Verification items for the finished model (mm, model axes). Face numbers are marked on the shaded views. Round coordinates to 2 decimals unless told otherwise and drop trailing zeros. Write each loop counter-clockwise with the first axis right and the second up, starting at its lowest first coordinate (ties: lowest second). Pieces come first, ordered by that corner, then holes.
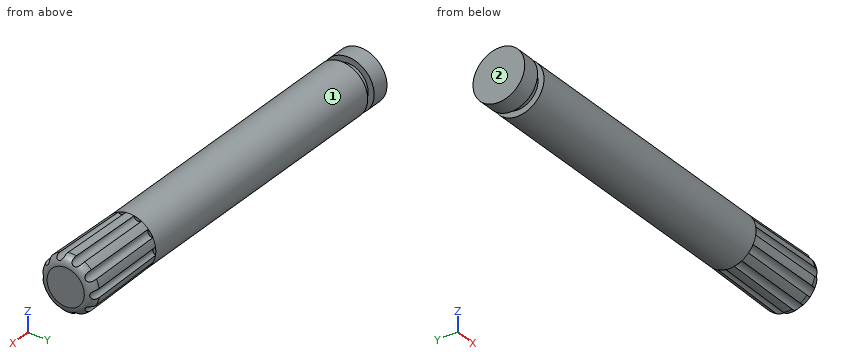
from build123d import *

# Parameters (mm, degrees)
SKETCH1_R                = 1.5
EXTRUDE1_DEPTH           = 18
EXTRUDE1_OTHER_WAY_DEPTH = 5
EXTRUDE1_OTHER_WAY_TAPER = -1
FILLET1_R                = 0.5
SKETCH2_R                = 0.25
CUT_EXTRUDE1_DEPTH       = 5
CIRPATTERN1_COUNT        = 10
SKETCH3_W                = 0.5
SKETCH3_H                = 0.930924855


with BuildPart() as part:
    # Sketch1 → Extrude1 (new body)
    with BuildSketch(Plane(origin=(0, 0, 0), x_dir=(0, 0, -1), z_dir=(1, 0, 0))):
        Circle(SKETCH1_R)
    extrude(amount=-EXTRUDE1_DEPTH)

    # Sketch1 → Extrude1 other way (add)
    with BuildSketch(Plane(origin=(0, 0, 0), x_dir=(0, 0, -1), z_dir=(1, 0, 0))):
        Circle(SKETCH1_R)
    extrude(amount=EXTRUDE1_OTHER_WAY_DEPTH, taper=EXTRUDE1_OTHER_WAY_TAPER)

    # Fillet1
    fillet1_edges = [part.edges().sort_by_distance(p)[0] for p in [
        (5, 0, 1.587275325),
    ]]
    fillet(fillet1_edges, radius=FILLET1_R)

    # Sketch2 → Cut-Extrude1 (cut)
    with BuildSketch(Plane(origin=(5, 0, 0), x_dir=(0, 0, -1), z_dir=(1, 0, 0))):
        with Locations((0, 1.587275325)):
            Circle(SKETCH2_R)
    cut_extrude1 = extrude(amount=-CUT_EXTRUDE1_DEPTH, mode=Mode.SUBTRACT)

    # CirPattern1: Cut-Extrude1 ×10 about axis
    cirpattern1_axis = Axis((0, 0, 0), (1, 0, 0))
    for i in range(1, CIRPATTERN1_COUNT):
        add(cut_extrude1.rotate(cirpattern1_axis, i * 360 / CIRPATTERN1_COUNT), mode=Mode.SUBTRACT)

    # Sketch3 → Cut-Revolve2 (revolve, cut)
    with BuildSketch(Plane.XY):
        with Locations((-16.75, 1.615462428)):
            Rectangle(SKETCH3_W, SKETCH3_H)
    revolve(axis=Axis((-18, 0, 0), (1, 0, 0)), mode=Mode.SUBTRACT)


solid = part.part
Q1. Sectioned sample at A-A (z = 0). Enter the section's corners in (x, y).
Recorded:
outline: (-18, -1.5) - (-17, -1.5) - (-17, -1.15) - (-16.5, -1.15) - (-16.5, -1.5) - (0, -1.5) - (0, -1.34) - (4.93, -1.34) arc R0.5 ccw to (5, -1.08) - (5, 1.08) arc R0.5 ccw to (4.93, 1.34) - (0, 1.34) - (0, 1.5) - (-16.5, 1.5) - (-16.5, 1.15) - (-17, 1.15) - (-17, 1.5) - (-18, 1.5) - close
Q2. Release check for a two-part mould opening along Y. For the marked faces 1 and 2 record: released by +Y, released by -Y, zero draft, split by the parting line, or undercut.
Recorded:
face 1: split by the parting line
face 2: zero draft
Q3. Sectioned sample at B-B (x = 3.25). Enter the section's corners in (y, z), plus the area to 3 significant figures.
Recorded:
outline: (-1.54, -0.24) arc R1.56 ccw to (-1.39, -0.71) arc R0.25 cw to (-1.1, -1.1) arc R1.56 ccw to (-0.71, -1.39) arc R0.25 cw to (-0.24, -1.54) arc R1.56 ccw to (0.24, -1.54) arc R0.25 cw to (0.71, -1.39) arc R1.56 ccw to (1.1, -1.1) arc R0.25 cw to (1.39, -0.71) arc R1.56 ccw to (1.54, -0.24) arc R0.25 cw to (1.54, 0.24) arc R1.56 ccw to (1.39, 0.71) arc R0.25 cw to (1.1, 1.1) arc R1.56 ccw to (0.71, 1.39) arc R0.25 cw to (0.24, 1.54) arc R1.56 ccw to (-0.24, 1.54) arc R0.25 cw to (-0.71, 1.39) arc R1.56 ccw to (-1.1, 1.1) arc R0.25 cw to (-1.39, 0.71) arc R1.56 ccw to (-1.54, 0.24) arc R0.25 cw to start
area: 6.82 mm2
Q4. Material ranges on line 1 along Z through (x, y) = (2.5, -0.5); line 2 along Y through (x, z) = (0.5, -1.1); line 3 along Y through (x, z) = (3, -0.65), recorded low to high.
Recorded:
line 1: z = -1.26 to 1.26
line 2: y = -1.03 to 1.03
line 3: y = -1.41 to 1.41
Q5. Sectioned sample at C-C (x = -9.75). Enter the section's corners in (y, z), plus the area to 3 significant figures.
Recorded:
outline: circle Ø3 at (0, 0)
area: 7.07 mm2
Q6. Depth check by flat-ended pin: P1, Ø1, axis at x = -2.5, y = 0.5, coming from the +Z side; P2, Ø1, axis at x = 2.5, z = -0.5, coming from the +Y side. Enter the tip coordinate at first touch or a pass-through.
Recorded:
P1: stops at z = 1.5
P2: stops at y = 1.53
